CAD build for the part. Positions are in the model's coordinates, mm. A direction names the side the tool comes from. Coordinates: 2 decimals unless noted, no trailing zeros. Order: outer loops, then holes, each group sorted by start corner. A loop starts at its lowest first (then second) coordinate and runs counter-clockwise, first axis right, second up. Notation, with made-up numbers: M 52.5,-5.5 L 78.5,-5.5 A32 cw 78.5,25.5 Z; hole C 52.25,49 d5. An arc over 180 degrees is marked long. Write item = value, one per line. Start each with the question number.
```python
from build123d import *

# Parameters (mm, degrees)
ESQUISSE1_W             = 130
ESQUISSE1_H             = 130
BASE_EXTRUSION_DEPTH    = 105
ENL_V_MAT_EXTRU_1_DEPTH = 115
ESQUISSE4_R             = 2.5
ENL_V_MAT_EXTRU_2_DEPTH = 5


with BuildPart() as part:
    # Esquisse1 → Base-Extrusion (new body)
    with BuildSketch(Plane(origin=(0, 0, 0), x_dir=(0, 0, -1), z_dir=(1, 0, 0))):
        with Locations((65, 65)):
            Rectangle(ESQUISSE1_W, ESQUISSE1_H)
    extrude(amount=BASE_EXTRUSION_DEPTH)

    # Esquisse3 → Enlèv. mat.-Extru.1 (cut)
    with BuildSketch(Plane.XY.offset(-10)):
        Polygon((0, 0), (20, 0), (0, 20), align=None)
        Polygon((0, 130), (0, 110), (20, 130), align=None)
        Polygon((105, 130), (105, 110), (85, 130), align=None)
        Polygon((105, 0), (105, 20), (85, 0), align=None)
    extrude(amount=-ENL_V_MAT_EXTRU_1_DEPTH, mode=Mode.SUBTRACT)

    # Esquisse4 → Enlèv. mat.-Extru.2 (cut)
    with BuildSketch(Plane(origin=(0, 0, -130), x_dir=(-1, 0, 0), z_dir=(0, 0, -1))):
        with Locations((-6, 124)):
            Circle(ESQUISSE4_R)
        with Locations((-99, 124)):
            Circle(ESQUISSE4_R)
    extrude(amount=-ENL_V_MAT_EXTRU_2_DEPTH, mode=Mode.SUBTRACT)


solid = part.part
```
1. Slice it at B-B (y = 124). Write the cut outline in (x, z).
2. Probe L1, parallel to Y at x = 99, z = -128.85; L2, parallel to X at y = 11.5, z = -18; L3, parallel to X at y = 16.5, z = -122.5. List the from-to ranges inside material, lowest first.
3. 3-axis set-ups, long thin cutter, end or side, ignore diameter. For faces 5 (the flat face through (99, 6, -125)), 6 (the flat face through (97, 122, -10)), 7 (the cylindrical face through (99.33, 126.48, -127.54)), 8 (the flat face through (5, 6, -125)), 9 (the flat face through (10, 120, -67)): which of +Z, -Z, +X, -X, +Y, -Y reach the whole face in a straight line?
4. Slice it at A-A (x = 99). Write the cut outline in (y, z), plus the area to 3 significant figures.
5. Flat gauge pins, fed straight in: pin 1 (5 mm diameter, centred on x = 94, z = -106, fed in from +Y); pin 2 (1 mm diameter, centred on x = 18.5, z = -25, fed in from +Y). Where does each tip first touch, or does it go through?
6. Slice it at D-D (y = 18). Write the cut outline in (x, z).
7. Mould opens along Y. For faces 1 (the flat face through (0, 66, -64)), 2 (the cylindrical face through (6.33, 126.48, -127.54)), 3 (the flat face through (95, 10, -67)), 4 (the flat face through (52, 130, -64)) say: released by +Y, released by -Y, zero draft, split by the parting line, or undercut.
8. Slice it at C-C (z = -86). Write the cut outline in (x, y).
Calculated:
q1.outline = M 0,-130 L 3.5,-130 L 3.5,-125 L 0,-125 Z; M 0,-10 L 14,-10 L 14,-125 L 8.5,-125 L 8.5,-130 L 96.5,-130 L 96.5,-125 L 91,-125 L 91,-10 L 105,-10 L 105,0 L 0,0 Z; M 101.5,-130 L 105,-130 L 105,-125 L 101.5,-125 Z
q2.L1 = 0 to 121.5, 126.5 to 130
q2.L2 = 8.5 to 96.5
q2.L3 = 3.5 to 101.5
q3.face_5 = +X, -Y
q3.face_6 = +X, +Y
q3.face_7 = -Z
q3.face_8 = -X, -Y
q3.face_9 = -X, +Y
q4.outline = M 0,-130 L 121.5,-130 L 121.5,-125 L 116,-125 L 116,-10 L 130,-10 L 130,0 L 0,0 L 0,-10 L 14,-10 L 14,-125 L 0,-125 Z; M 126.5,-130 L 130,-130 L 130,-125 L 126.5,-125 Z
q4.area = 13,700 mm²
q5.pin_1 = 123.5
q5.pin_2 = 129
q6.outline = M 0,-130 L 105,-130 L 105,-125 L 103,-125 L 103,-10 L 105,-10 L 105,0 L 0,0 L 0,-10 L 2,-10 L 2,-125 L 0,-125 Z
q7.face_1 = zero draft
q7.face_2 = undercut
q7.face_3 = released by -Y
q7.face_4 = released by +Y
q8.outline = M 0,20 L 20,0 L 85,0 L 105,20 L 105,110 L 85,130 L 20,130 L 0,110 Z
